Input: part model. Units: mm. Frame: model coordinates. Face numbers are marked on the shaded views. A direction names the side the tool comes from. Round coordinates to 2 decimals unless told otherwise and drop trailing zeros. Write each loop counter-clockwise with the first axis right and the second up, starting at its lowest first coordinate (ties: lowest second). Pieces come first, ordered by that corner, then holes. Notation, with made-up numbers: M 88,-26 L 100,-26 A7 cw 100,-22 Z; hole C 47,-2 d4. An arc over 180 degrees is marked long. Answer as CSV lines item,"result". Start each with the question number.
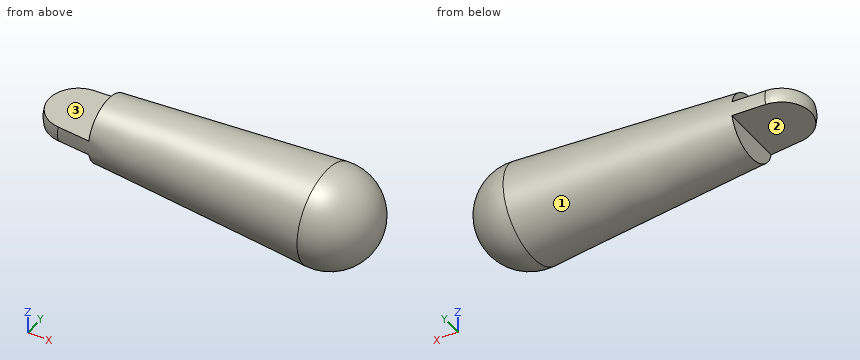
```python
from build123d import *

# Parameters (mm, degrees)
CUT_EXTRUDE2_DEPTH      = 157.48
CUT_EXTRUDE2_DEPTH_BACK = 157.48
SKETCH2_W               = 101.6
SKETCH2_H               = 127


with BuildPart() as part:
    # Sketch1 → Revolve1 (revolve)
    with BuildSketch(Plane.XY):
        with BuildLine():
            Line((-213.36, 0), (213.36, 0))
            Line((213.36, 0), (294.64, 0))
            ThreePointArc((294.64, 0), (268.742984494, 59.490868447), (207.554285714, 81.072387911))
            Line((207.554285714, 81.072387911), (-216.988571429, 50.670242445))
            ThreePointArc((-216.988571429, 50.670242445), (-250.541792779, 34.614365309), (-264.16, 0))
            Line((-264.16, 0), (-213.36, 0))
        make_face()
    revolve(axis=Axis((-213.36, 0, 0), (1, 0, 0)))

    # Sketch2 → Cut-Extrude2 (cut, two sides: drawn at the far end of the back side and taken through both)
    with BuildSketch(Plane(origin=(0, 0, 0), x_dir=(1, 0, 0), z_dir=(0, 1, 0)).offset(-CUT_EXTRUDE2_DEPTH_BACK)):
        with Locations((-213.36, 76.2)):
            Rectangle(SKETCH2_W, SKETCH2_H)
        with Locations((-213.36, -76.2)):
            Rectangle(SKETCH2_W, SKETCH2_H)
    extrude(amount=CUT_EXTRUDE2_DEPTH + CUT_EXTRUDE2_DEPTH_BACK, mode=Mode.SUBTRACT)


solid = part.part
```
Item 1: Line query: line 1 (Z direction, x = -242, y = 22.5); line 2 (Z direction, x = -83, y = -28.5); line 3 (Y direction, x = -90.5, z = -37.5). Output: solid intervals per line, ascending. Write a range as [from, to].
Item 2: Cut plane A-A, the plane y = 0. Return loops of the section in (x, z), plus the area to 3 significant figures.
Item 3: Cut plane C-C, the plane x = 168. Return loops of the section in (y, z), plus the area to 3 significant figures.
Item 4: Cut plane B-B, the plane z = 0. Return loops of the section in (x, y), plus the area to 3 significant figures.
Item 5: Cut plane D-D, the plane x = -64.5. Return loops of the section in (y, z), plus the area to 3 significant figures.
Item 6: Access query for the marked faces 1, 2 and 3. Directions: +Z, -Z, +X, -X, +Y, -Y. A direction counts if a zero-diameter tool reaches every point of the face in a straight line with its end or side. Return the directions, or none.
Item 7: Pin query (flat end, axial travel): pin 1 Ø6 at (x, z) = (113, 27) entering from -Y; pin 2 Ø12.5 at (y, z) = (-12.5, -26) entering from -X; pin 3 Ø5 at (x, y) = (-66.5, -59.5) entering from -Z; pin 4 Ø10 at (x, y) = (-135, 64.5) entering from +Z. Return the tip coordinate at first contact, or that it passes through.
Results list:
1,line 1,"[-12.7, 12.7]"
1,line 2,"[-53.1, 53.1]"
1,line 3,"[-46.49, 46.49]"
2,outline,"M -262.55,-12.7 L -162.56,-12.7 L -162.56,-54.57 L 207.55,-81.07 A81.28 ccw long 207.55,81.07 L -162.56,54.57 L -162.56,12.7 L -262.55,12.7 A50.8 ccw Z"
2,area,"64,100 mm²"
3,outline,"C 0,0 d156.48"
3,area,"19,200 mm²"
4,outline,"M -216.99,-50.67 L 207.55,-81.07 A81.28 ccw long 207.55,81.07 L -216.99,50.67 A50.8 ccw Z"
4,area,"70,900 mm²"
5,outline,"C 0,0 d123.18"
5,area,"11,900 mm²"
6,face 1,"-X"
6,face 2,"-Z, -X, +Y, -Y"
6,face 3,"+Z, -X, +Y, -Y"
7,pin 1,"y = -70.34"
7,pin 2,"x = -162.56"
7,pin 3,"z = -22.97"
7,pin 4,"through"
